Autodesk Inventor part; units mm, degrees
ref_plane "YZ Plane" through (0, 0, 0) normal (1, 0, 0) x (0, 1, 0)
ref_plane "XZ Plane" through (0, 0, 0) normal (0, 1, 0) x (-1, 0, 0)
ref_plane "XY Plane" through (0, 0, 0) normal (0, 0, 1) x (1, 0, 0)
sketch "Sketch1" plane through (0, 0, 0) normal (0, 0, 1) x (1, 0, 0)
  line L0 (0, 0) -> (25.4, 0)
  line L1 (25.4, 0) -> (25.4, 63.5)
  line L2 (25.4, 63.5) -> (0, 63.5)
  line L3 (0, 63.5) -> (0, 0)
  circle A0 centre (12.7, 50.8) radius 3.3782
  circle A1 centre (12.7, 12.7) radius 3.3782
  dimension "d0" = 25.4
  dimension "d1" = 63.5
  dimension "d2" = 6.7564
  dimension "d3" = 6.7564
  dimension "d4" = 12.7
  dimension "d5" = 12.7
  dimension "d6" = 12.7
  dimension "d7" = 12.7
extrude "Plate1" add sketch "Sketch1" along normal blind 3.175
sketch "Sketch2" plane through (26.67, 63.5, 4.445) normal (1, 0, 0) x (0, 1, 0)
  line L0 (-63.5, 0) -> (0, 0)
  line L1 (0, 0) -> (0, 20.955)
  line L2 (0, 20.955) -> (-63.5, 20.955)
  line L3 (-63.5, 20.955) -> (-63.5, 0)
edge flange "Flange1" height 25.4 angle 90 thickness 3.175 bend radius 1.27 thickness toward (1, 0, 0) relief tear relief width 3.175 relief depth 1.5875 edges at (25.4, 31.75, 3.175) wall of the first edge with corners at (26.67, 0, 4.445) (26.67, 63.5, 4.445) (26.67, 63.5, 25.4) (26.67, 0, 25.4)
bend "Bend1"
corner "Corner1"
sketch "Sketch3" plane through (29.845, 0, 25.4) normal (1, 0, 0) x (0, 0, -1)
  line L0 (0, 63.5) -> (20.955, 63.5)
  line L1 (0, 0) -> (0, 63.5)
  line L2 (20.955, 0) -> (0, 0)
  circle A0 centre (6.35, 31.75) radius 1.5875
  line L3 (0, 38.1) -> (20.955, 63.5)
  line L4 (0, 25.4) -> (20.955, 0)
  point P0 (25.4, 0)
  dimension "d19" = 3.175
  dimension "d20" = 6.35
  dimension "d21" = 31.75
  dimension "d22" = 12.7
  dimension "d23" = 25.4
sketch "Sketch4" plane through (-1.27, 0, 4.445) normal (-1, 0, 0) x (0, -1, 0)
  line L0 (-63.5, 0) -> (0, 0)
  line L1 (0, 0) -> (0, 20.955)
  line L2 (0, 20.955) -> (-63.5, 20.955)
  line L3 (-63.5, 20.955) -> (-63.5, 0)
edge flange "Flange2" height 25.4 angle 90 thickness 3.175 bend radius 1.27 thickness toward (-1, 0, 0) relief tear relief width 3.175 relief depth 1.5875 edges at (0, 31.75, 3.175) wall of the first edge with corners at (-1.27, 63.5, 4.445) (-1.27, 0, 4.445) (-1.27, 0, 25.4) (-1.27, 63.5, 25.4)
bend "Bend2"
corner "Corner2"
extrude "Extrusion1" cut sketch "Sketch3" against normal blind 76.2
equation "\"d9\" = BendReliefWidth"
equation "\"d10\" = BendReliefDepth"
equation "\"d11\" = MinimumRemnant"
equation "\"d12\" = BendRadius"
equation "\"d16\" = CornerReliefSize"
equation "\"d17\" = GapSize"
equation "\"d18\" = JacobiRadiusSize"
equation "\"d26\" = BendReliefWidth"
equation "\"d27\" = BendReliefDepth"
equation "\"d28\" = MinimumRemnant"
equation "\"d29\" = BendRadius"
equation "\"d33\" = CornerReliefSize"
equation "\"d34\" = GapSize"
equation "\"d35\" = JacobiRadiusSize"
equation "\"BendRadius\" = Thickness"
equation "\"BendReliefWidth\" = Thickness"
equation "\"BendReliefDepth\" = 0.5 * Thickness"
equation "\"CornerReliefSize\" = 4 * Thickness"
equation "\"MinimumRemnant\" = 2 * Thickness"
equation "\"TransitionRadius\" = BendRadius"
equation "\"JacobiRadiusSize\" = BendRadius"
equation "\"GapSize\" = Thickness"
equation "\"d8\" = BendRadius"
properties part number "BackPistonHinge-Tower"
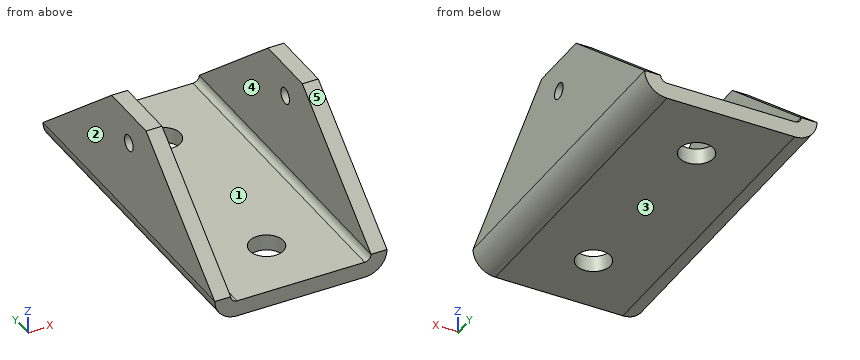
CAD build for the part. Positions are in the model's coordinates, mm. Face numbers are marked on the shaded views. A direction names the side the tool comes from. Coordinates: 2 decimals unless noted, no trailing zeros. Order: outer loops, then holes, each group sorted by start corner. A loop starts at its lowest first (then second) coordinate and runs counter-clockwise, first axis right, second up. Notation, with made-up numbers: M 44,21 L 89,21 A10 cw 89,32 Z; hole C -37,-17.75 d5. An arc over 180 degrees is marked long. Write each question's results on one line, items separated by ' | '. Start each with the question number.
Q1. Which spindle directions (+Z, -Z, +X, -X, +Y, -Y) get a long thin tool onto all of the face, cutting with end or side? Do the marked faces 4 and 5. Say none if no direction does.
Q2. Cut at C-C (z = 19.05). List the corners of the cut face in (x, y) (1 decimal), then the cut area to 3 significant figures.
Q3. Drill centre lines: probe 1 along Y at (x, z) = (12.7, 0.8); probe 2 along X at (y, z) = (31, 22) (3 decimals); probe 3 along Y at (x, z) = (15.5, 1.5). Where is each one in solid material? Low to high. Write a range as from..to.
Q4. Cut at A-A (x = 12.7). List the corners of the cut face in (y, z) (3 decimals).
Q5. Pull direction X, two halves, no side cores. Call the marked faces 1, 2 and 3: +X half, -X half, draft (parallel to the pull), parting line (faces both ways), or undercut.
Q6. Cut at D-D (z = 12.5). List the corners of the cut face in (x, y) (3 decimals), then the cut area to 3 significant figures.
Q7. Flat gauge pins, fed straight in: P1, Ø2, axis at x = 13, z = 4, coming from the -Y side; P2, Ø9, axis at x = 12.7, y = 12.7, coming from the +Z side (3 decimals). Where does each tip first touch, or does it go through?
Q8. Cut at B-B (y = 31.75). List the corners of the cut face in (x, z) (1 decimal), then the cut area to 3 significant figures.
Found:
1) face 4: +Z, +Y, -Y | face 5: +Z, +X, -X, -Y
2) outline: M -4.4,17.7 L -1.3,17.7 L -1.3,30.2 L -4.4,30.2 Z; M -4.4,33.3 L -1.3,33.3 L -1.3,45.8 L -4.4,45.8 Z; M 26.7,17.7 L 29.8,17.7 L 29.8,30.2 L 26.7,30.2 Z; M 26.7,33.3 L 29.8,33.3 L 29.8,45.8 L 26.7,45.8 Z | area: 158 mm²
3) probe 1: 0..9.32, 16.08..47.42, 54.18..63.5 | probe 2: -4.445..-1.27, 26.67..29.845 | probe 3: 0..10.81, 14.59..48.91, 52.69..63.5
4) outline: M 0,0 L 9.322,0 L 9.322,3.175 L 0,3.175 Z; M 16.078,0 L 47.422,0 L 47.422,3.175 L 16.078,3.175 Z; M 54.178,0 L 63.5,0 L 63.5,3.175 L 54.178,3.175 Z
5) face 1: undercut | face 2: -X half | face 3: draft
6) outline: M -4.445,9.764 L -1.27,9.764 L -1.27,53.736 L -4.445,53.736 Z; M 26.67,9.764 L 29.845,9.764 L 29.845,53.736 L 26.67,53.736 Z | area: 279 mm²
7) P1: y = 0 | P2: z = 3.175
8) outline: M -4.4,4.4 A4.4 ccw 0,0 L 25.4,0 A4.4 ccw 29.8,4.4 L 29.8,17.5 L 26.7,17.5 L 26.7,4.4 A1.3 cw 25.4,3.2 L 0,3.2 A1.3 cw -1.3,4.4 L -1.3,17.5 L -4.4,17.5 Z; M -4.4,20.6 L -1.3,20.6 L -1.3,25.4 L -4.4,25.4 Z; M 26.7,20.6 L 29.8,20.6 L 29.8,25.4 L 26.7,25.4 Z | area: 222 mm²
